Could you check a few things on this model? Use its own coordinates, in mm. Face numbers are marked on the shaded views. Round coordinates to 2 decimals unless told otherwise and drop trailing zeros. Write each loop counter-clockwise with the first axis right and the second up, starting at its lowest first coordinate (ties: lowest second). Pieces come first, ordered by that corner, then holes. Notation, with made-up numbers: (41.25, 0.5) -> (83.25, 0.5) arc R7 ccw to (83.25, 7.5) -> close; hole circle Ø8 at (85, 81.5). An arc over 180 degrees is marked (long way). Answer in a Markdown table with one row per item.
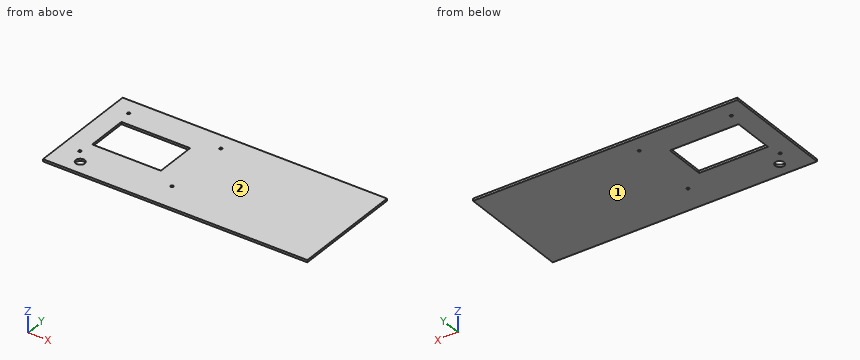
from build123d import *

# Parameters (mm, degrees)
SKETCH_1_W      = 350
SKETCH_1_H      = 150
SKETCH_1_R      = 1.75
SKETCH_1_R_2    = 6
SKETCH_1_W_2    = 91
SKETCH_1_H_2    = 55
EXTRUDE_1_DEPTH = 3


with BuildPart() as part:
    # 草图1 → 凸台-拉伸1 (new body)
    with BuildSketch(Plane.XY):
        with Locations((0, 75)):
            Rectangle(SKETCH_1_W, SKETCH_1_H)
        with Locations((-151.652414134, 128.095526692)):
            Circle(SKETCH_1_R, mode=Mode.SUBTRACT)
        with Locations((-29.652414134, 128.095526692)):
            Circle(SKETCH_1_R, mode=Mode.SUBTRACT)
        with Locations((-29.652414134, 36.095526692)):
            Circle(SKETCH_1_R, mode=Mode.SUBTRACT)
        with Locations((-151.652414134, 36.095526692)):
            Circle(SKETCH_1_R, mode=Mode.SUBTRACT)
        with Locations((-139, 19)):
            Circle(SKETCH_1_R_2, mode=Mode.SUBTRACT)
        with Locations((-102.777414134, 82.095526692)):
            Rectangle(SKETCH_1_W_2, SKETCH_1_H_2, mode=Mode.SUBTRACT)
    extrude(amount=EXTRUDE_1_DEPTH)


solid = part.part
1) Imagine slicing it at C-C, the plane x = -101. Please give me the cut outline in (y, z).
Findings:
| item | result |
|---|---|
| outline | (0, 0) -> (54.6, 0) -> (54.6, 3) -> (0, 3) -> close; (109.6, 0) -> (150, 0) -> (150, 3) -> (109.6, 3) -> close |
2) Please list where these lines run through material, in increasing order: line 1 (Y direction, x = -139, z = 1.45); line 2 (Y direction, x = -118, z = 1.25); line 3 (X direction, y = 72, z = 0.4).
Findings:
| item | result |
|---|---|
| line 1 | y = 0 to 13, 25 to 54.6, 109.6 to 150 |
| line 2 | y = 0 to 54.6, 109.6 to 150 |
| line 3 | x = -175 to -148.28, -57.28 to 175 |
3) Imagine slicing it at A-A, the plane y = 103. Please give me the cut outline in (x, z), plus the area to 3 significant figures.
Findings:
| item | result |
|---|---|
| outline | (-175, 0) -> (-148.28, 0) -> (-148.28, 3) -> (-175, 3) -> close; (-57.28, 0) -> (175, 0) -> (175, 3) -> (-57.28, 3) -> close |
| area | 777 mm^2 |
4) Imagine slicing it at B-B, the plane x = -139. Please give me the cut outline in (y, z), plus the area to 3 significant figures.
Findings:
| item | result |
|---|---|
| outline | (0, 0) -> (13, 0) -> (13, 3) -> (0, 3) -> close; (25, 0) -> (54.6, 0) -> (54.6, 3) -> (25, 3) -> close; (109.6, 0) -> (150, 0) -> (150, 3) -> (109.6, 3) -> close |
| area | 249 mm^2 |
5) For pin 1 (19 mm diameter, centred on x = -139, y = 19, fed in from -Z); pin 2 (3 mm diameter, centred on x = -29.65, y = 36.1, fed in from +Z), each with a flat end and sliding along its axis, tell me the tip position at first contact or that it passes through.
Findings:
| item | result |
|---|---|
| pin 1 | stops at z = 0 |
| pin 2 | passes through |
6) Imagine slicing it at D-D, the plane z = 2.2. Please give me the cut outline in (x, y).
Findings:
| item | result |
|---|---|
| outline | (-175, 0) -> (175, 0) -> (175, 150) -> (-175, 150) -> close; hole circle Ø3.5 at (-151.65, 36.1); hole circle Ø3.5 at (-151.65, 128.1); hole (-148.28, 54.6) -> (-57.28, 54.6) -> (-57.28, 109.6) -> (-148.28, 109.6) -> close; hole circle Ø12 at (-139, 19); hole circle Ø3.5 at (-29.65, 36.1); hole circle Ø3.5 at (-29.65, 128.1) |
7) Thinking about a two-plate mould opening in Z: for the marked faces 1 and 2, which applies, +Z half, -Z half, draft (parallel to the pull), parting line (faces both ways), or undercut?
Findings:
| item | result |
|---|---|
| face 1 | -Z half |
| face 2 | +Z half |
